```python
from build123d import *

# Parameters (mm, degrees)
SKETCH1_W           = 40
SKETCH1_H           = 20
BOSS_EXTRUDE1_DEPTH = 2
SKETCH2_W           = 35.84
SKETCH2_H           = 15.84
BOSS_EXTRUDE2_DEPTH = 10
SKETCH4_W           = 30.84
SKETCH4_H           = 10.84
CUT_EXTRUDE1_DEPTH  = 10
FILLET1_R           = 2


with BuildPart() as part:
    # Sketch1 → Boss-Extrude1 (new body)
    with BuildSketch(Plane.XY):
        Rectangle(SKETCH1_W, SKETCH1_H)
    extrude(amount=BOSS_EXTRUDE1_DEPTH)

    # Sketch2 → Boss-Extrude2 (add)
    with BuildSketch(Plane.XY.offset(2)):
        Rectangle(SKETCH2_W, SKETCH2_H)
    extrude(amount=BOSS_EXTRUDE2_DEPTH)

    # Sketch4 → Cut-Extrude1 (cut)
    with BuildSketch(Plane.XY.offset(12)):
        Rectangle(SKETCH4_W, SKETCH4_H)
    extrude(amount=-CUT_EXTRUDE1_DEPTH, mode=Mode.SUBTRACT)

    # Fillet1
    fillet1_edges = [part.edges().sort_by_distance(p)[0] for p in [
        (-15.42, 0, 2),
        (-15.42, -5.42, 7),
        (0, -5.42, 2),
        (15.42, -5.42, 7),
        (15.42, 0, 2),
        (15.42, 5.42, 7),
        (0, 5.42, 2),
        (-15.42, 5.42, 7),
    ]]
    fillet(fillet1_edges, radius=FILLET1_R)


solid = part.part
```
Could you check a few things on this model? Use its own coordinates, in mm. A direction names the side the tool comes from. Round coordinates to 2 decimals unless told otherwise and drop trailing zeros. Write each loop counter-clockwise with the first axis right and the second up, starting at its lowest first coordinate (ties: lowest second). Pieces come first, ordered by that corner, then holes. Notation, with made-up numbers: M 43,-4 L 57,-4 A19 cw 57,11 Z; hole C 18.25,-29.75 d4. An arc over 180 degrees is marked long. Write each question's results on one line, items separated by ' | '. Start each with the question number.
1. I'm going to push flat-ended pins straight in: pin 1 Ø2 at (y, z) = (-0.5, 9) entering from -X; pin 2 Ø6.5 at (x, z) = (5.5, 6.5) entering from -Y; pin 3 Ø2 at (x, y) = (4.5, 1) entering from +Z. Where does each tip first touch, or does it pass through?
2. Imagine slicing it at B-B on y = 1.5. List the corners of the cut face in (x, z) for me.
3. Imagine slicing it at D-D on x = -10.5. List the corners of the cut face in (y, z) for me, and give its area (3 significant figures).
4. I need wall thicknesses on L1, parallel to Y at x = 0, z = 9.5; L2, parallel to X at y = 3, z = 4.5; L3, parallel to Z at x = -12.5, y = -2. Which ranges of each line are inside material? Lowest first, please. Write a range as from..to.
5. Imagine slicing it at C-C on x = 17.5. List the corners of the cut face in (y, z) for me, and give its area (3 significant figures).
6. Thinking about a two-plate mould opening in X: for faces 1 (the face through (-17.92, 0, 7)), 2 (the face through (-1.6, -8.1, 2)), 3 (the face through (0, -5.42, 8)), which applies, +X half, -X half, draft (parallel to the pull), parting line (faces both ways), or undercut?
7. On a 3-axis mill with a long thin cutter (end or side, diameter ignored), from which of +Z, -Z, +X, -X, +Y, -Y can I reach the whole of each face in a straight line? I mean faces 4 (the face through (0, -10, 1)), 5 (the face through (0.19, 4.85, 2.6)), 6 (the face through (0, 7.92, 7)), 7 (the face through (17.92, 0, 7)), 8 (the face through (0, -7.92, 7)). Say none if no direction works.
8. Imagine slicing it at A-A on z = 7.5. List the corners of the cut face in (x, y) for me, and give its area (3 significant figures).
Result sheet:
1) pin 1: stops at x = -17.92 | pin 2: stops at y = -7.92 | pin 3: stops at z = 2
2) outline: M -20,0 L 20,0 L 20,2 L 17.92,2 L 17.92,12 L 15.42,12 L 15.42,4 A2 cw 13.42,2 L -13.42,2 A2 cw -15.42,4 L -15.42,12 L -17.92,12 L -17.92,2 L -20,2 Z
3) outline: M -10,0 L 10,0 L 10,2 L 7.92,2 L 7.92,12 L 5.42,12 L 5.42,4 A2 cw 3.42,2 L -3.42,2 A2 cw -5.42,4 L -5.42,12 L -7.92,12 L -7.92,2 L -10,2 Z | area: 91.7 mm^2
4) L1: y = -7.92..-5.42, 5.42..7.92 | L2: x = -17.92..-15.42, 15.42..17.92 | L3: z = 0..2
5) outline: M -10,0 L 10,0 L 10,2 L 7.92,2 L 7.92,12 L -7.92,12 L -7.92,2 L -10,2 Z | area: 198 mm^2
6) face 1: -X half | face 2: draft | face 3: undercut
7) face 4: +Z, -Z, +X, -X, -Y | face 5: +Z | face 6: +Z, +X, -X, +Y | face 7: +Z, +X, +Y, -Y | face 8: +Z, +X, -X, -Y
8) outline: M -17.92,-7.92 L 17.92,-7.92 L 17.92,7.92 L -17.92,7.92 Z; hole M -15.42,-3.42 A2 ccw -13.42,-5.42 L 13.42,-5.42 A2 ccw 15.42,-3.42 L 15.42,3.42 A2 ccw 13.42,5.42 L -13.42,5.42 A2 ccw -15.42,3.42 Z | area: 237 mm^2
